Autodesk Inventor part; units mm, degrees
ref_plane "YZ Plane" through (0, 0, 0) normal (1, 0, 0) x (0, 1, 0)
ref_plane "XZ Plane" through (0, 0, 0) normal (0, 1, 0) x (-1, 0, 0)
ref_plane "XY Plane" through (0, 0, 0) normal (0, 0, 1) x (1, 0, 0)
sketch "Sketch1" plane through (0, 0, 0) normal (0, 1, 0) x (-1, 0, 0)
  circle A0 centre (0, 0) radius 4.5
  dimension "d0" = 9
extrude "Extrusion1" add sketch "Sketch1" along normal blind 28
sketch "Sketch2" plane through (0, 0, 0) normal (0, -1, 0) x (1, 0, 0)
  circle A0 centre (0, 0) radius 2.75
  dimension "d3" = 5.5
extrude "Extrusion2" add sketch "Sketch2" along normal blind 2
sketch "Sketch3" plane through (0, 28, 0) normal (0, 1, 0) x (1, 0, 0)
  circle A0 centre (0, 0) radius 2.75
  circle A1 centre (0, 0) radius 15
  dimension "d6" = 30
extrude "Extrusion3" add sketch "Sketch3" along normal blind 3 contours A0 | A1
properties part number "fsrTop"
Input: part model. Units: mm. Frame: model coordinates. A direction names the side the tool comes from. Coordinates: 2 decimals unless noted, no trailing zeros. Loops run counter-clockwise (first coordinate to the right, second up) from the corner with the lowest first, then second, coordinate; pieces in that order, holes last. Notation, with made-up numbers: M -22.5,49 L 8.5,49 A25 ccw 8.5,62 Z; hole C 58,24 d11. An arc over 180 degrees is marked long. Answer in a Markdown table with one row per item.
1. Reachability of faces 1 (the flat face through (0, 31, 0)), 2 (the cylindrical face through (-0.596, -0.986, 2.685)) from +Z, -Z, +X, -X, +Y, -Y: full face, straight path, thin tool, end or side. Return the list, or none.
Response:
| item | result |
|---|---|
| face 1 | +Z, -Z, +X, -X, +Y |
| face 2 | -Y |
2. Section C-C, the plane y = 7.5. Output: boundary loops of the cut face in (x, z).
Response:
| item | result |
|---|---|
| outline | C 0,0 d9 |
3. Section D-D, the plane z = 3.5. Output: boundary loops of the cut face in (x, y), then the cut area to 3 significant figures.
Response:
| item | result |
|---|---|
| outline | M -14.59,28 L -2.83,28 L -2.83,0 L 2.83,0 L 2.83,28 L 14.59,28 L 14.59,31 L -14.59,31 Z |
| area | 246 mm2 |
4. First-contact query: pin 1 (6 mm diameter, centred on y = 18, z = 3, fed in from +X); pin 2 (6 mm diameter, centred on x = -1.5, z = -7, fed in from -Y); pin 3 (3 mm diameter, centred on x = 1.5, y = 9.5, fed in from -Z). Flat tips, straight axial feed; report the tip coordinate or a pass-through.
Response:
| item | result |
|---|---|
| pin 1 | stops at x = 4.5 |
| pin 2 | stops at y = 0 |
| pin 3 | stops at z = -4.5 |
5. Section A-A, the plane z = 0. Output: boundary loops of the cut face in (x, y), then the cut area to 3 significant figures.
Response:
| item | result |
|---|---|
| outline | M -15,28 L -4.5,28 L -4.5,0 L -2.75,0 L -2.75,-2 L 2.75,-2 L 2.75,0 L 4.5,0 L 4.5,28 L 15,28 L 15,31 L -15,31 Z |
| area | 353 mm2 |
6. Section B-B, the plane x = 0. Output: boundary loops of the cut face in (y, z).
Response:
| item | result |
|---|---|
| outline | M -2,-2.75 L 0,-2.75 L 0,-4.5 L 28,-4.5 L 28,-15 L 31,-15 L 31,15 L 28,15 L 28,4.5 L 0,4.5 L 0,2.75 L -2,2.75 Z |
7. Material intervals for line 1 (Y direction, x = 7.5, z = 8.25); line 2 (Z direction, x = 0, y = 9); line 3 (Y direction, x = -1.25, z = -3), sorted ascending.
Response:
| item | result |
|---|---|
| line 1 | y = 28 to 31 |
| line 2 | z = -4.5 to 4.5 |
| line 3 | y = 0 to 31 |
